Read the model definition and answer for the solid it produces. Units are mm, in the model's axes. Face numbers are marked on the shaded views. A direction names the side the tool comes from. Round coordinates to 2 decimals unless told otherwise and drop trailing zeros. Write each loop counter-clockwise with the first axis right and the second up, starting at its lowest first coordinate (ties: lowest second). Pieces come first, ordered by that corner, then holes. Notation, with made-up numbers: (35, -12.5) - (52, -12.5) arc R18 ccw to (52, 19.5) - close; hole circle Ø6 at (-28.5, -9). An arc over 180 degrees is marked (long way). Use one line per item in the form item = value. Start each with the question number.
1) Each of these flat-tipped pins is pushed along its axis until it touches: pin 1 (2 mm diameter, centred on y = 28.5, z = 19.5, fed in from -X); pin 2 (1.5 mm diameter, centred on x = 23.5, y = 56.5, fed in from +Z); pin 3 (4 mm diameter, centred on x = 10, z = 11.5, fed in from +Y); pin 4 (6 mm diameter, centred on x = 8.5, z = -17, fed in from -Y). Where does it stop, or does it pass through?
2) For the marked faces 1 and 2, determine the directions among +Z, -Z, +X, -X, +Y, -Y from which every point of the face is accessible in a straight line to the end or side of a thin tool.
3) The part is cut by section B-B, the plane x = 0. Give the vertices of the cut face in (y, z).
4) Consider line 1 along X through (y, z) = (60, 0); line 2 along Y through (x, z) = (13, 12.5); line 3 along Z through (x, y) = (-3.5, 51.5). Determine where each line is inside the solid, lowest interval first. Write a range as from..to.
5) The part is cut by section C-C, the plane y = 36.5. Give the vertices of the cut face in (x, z).
6) The part is cut by section A-A, the plane z = 0. Give the vertices of the cut face in (x, y).
from build123d import *

# Parameters (mm, degrees)
SKETCH1_R           = 29.5
BOSS_EXTRUDE1_DEPTH = 86
CHAMFER1_SIZE       = 8
CHAMFER1_SIZE2      = 10
CHAMFER2_SIZE       = 2
CHAMFER2_SIZE2      = 8
SKETCH3_R           = 8.25
BOSS_EXTRUDE2_DEPTH = 2
SKETCH2_R           = 4
CUT_EXTRUDE1_DEPTH  = 98.388397666


with BuildPart() as part:
    # Sketch1 → Boss-Extrude1 (new body)
    with BuildSketch(Plane(origin=(0, 0, 0), x_dir=(1, 0, 0), z_dir=(0, 1, 0))):
        with Locations(Location((0, 0, 0), (0, 0, 270))):
            Circle(SKETCH1_R)
    extrude(amount=BOSS_EXTRUDE1_DEPTH)

    # Chamfer1
    chamfer1_edges = [part.edges().sort_by_distance(p)[0] for p in [
        (0, 86, -29.5),
    ]]
    chamfer1_side = [part.faces().sort_by_distance(p)[0] for p in [
        (0, 43, -29.5),
    ]]
    chamfer(chamfer1_edges, length=CHAMFER1_SIZE, length2=CHAMFER1_SIZE2, reference=chamfer1_side[0])

    # Chamfer2
    chamfer2_edges = [part.edges().sort_by_distance(p)[0] for p in [
        (0, 0, -29.5),
    ]]
    chamfer2_side = [part.faces().sort_by_distance(p)[0] for p in [
        (0, 0, 0),
    ]]
    chamfer(chamfer2_edges, length=CHAMFER2_SIZE, length2=CHAMFER2_SIZE2, reference=chamfer2_side[0])

    # Sketch3 → Boss-Extrude2 (add)
    with BuildSketch(Plane(origin=(0, 86, 0), x_dir=(1, 0, 0), z_dir=(0, 1, 0))):
        with Locations(Location((0, 0, 0), (0, 0, 270))):
            Circle(SKETCH3_R)
    extrude(amount=BOSS_EXTRUDE2_DEPTH)

    # Sketch2 → Cut-Extrude1 (cut, through all)
    with BuildSketch(Plane.XZ):
        with Locations(Location((0, 0, 0), (0, 0, 270))):
            Circle(SKETCH2_R)
    extrude(amount=-CUT_EXTRUDE1_DEPTH, mode=Mode.SUBTRACT)


solid = part.part
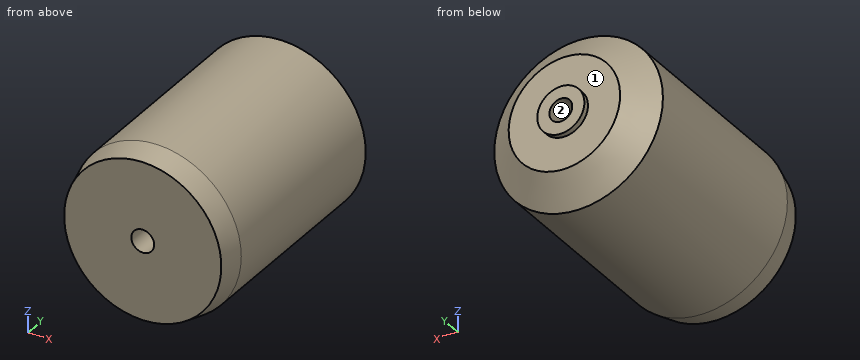
Geometry results:
q1.pin_1 = -22.98
q1.pin_2 = 18.78
q1.pin_3 = 86
q1.pin_4 = 0
q2.face_1 = +Y
q2.face_2 = +Y, -Y
q3.outline = (0, -27.5) - (8, -29.5) - (78, -29.5) - (86, -19.5) - (86, -8.25) - (88, -8.25) - (88, -4) - (0, -4) - close; (0, 4) - (88, 4) - (88, 8.25) - (86, 8.25) - (86, 19.5) - (78, 29.5) - (8, 29.5) - (0, 27.5) - close
q4.line_1 = -29.5..-4, 4..29.5
q4.line_2 = 0..86
q4.line_3 = -29.29..-1.94, 1.94..29.29
q5.outline = circle Ø59 at (0, 0); hole circle Ø8 at (0, 0)
q6.outline = (-29.5, 8) - (-27.5, 0) - (-4, 0) - (-4, 88) - (-8.25, 88) - (-8.25, 86) - (-19.5, 86) - (-29.5, 78) - close; (4, 0) - (27.5, 0) - (29.5, 8) - (29.5, 78) - (19.5, 86) - (8.25, 86) - (8.25, 88) - (4, 88) - close
